from build123d import *

# Parameters (mm, degrees)
CIRPATTERN2_COUNT = 3


with BuildPart() as part:
    # Sketch1 → Base-Revolve (revolve)
    with BuildSketch(Plane.XY):
        with BuildLine():
            Line((-50, 0), (-50, 1.25))
            ThreePointArc((-50, 1.25), (-49.010050505, 7.072345027), (-46.68190465, 12.5))
            Line((-46.68190465, 12.5), (46.650635095, 12.5))
            ThreePointArc((46.650635095, 12.5), (49.148145657, 6.470476128), (50, 0))
            Line((50, 0), (-50, 0))
        make_face()
    revolve(axis=Axis((-57, 0, 0), (1, 0, 0)))

    # Cut-Sweep3: sweep along a path in Sketch3
    with BuildLine(Plane(origin=(0, 0, 0), x_dir=(1, 0, 0), z_dir=(0, 1, 0))) as cut_sweep3_path:
        Line((-16.666666667, -12.5), (-10.416666667, -11.25))
        Line((-10.416666667, -11.25), (10.416666667, -11.25))
        Line((10.416666667, -11.25), (16.666666667, -12.5))
    # Sketch4 → Cut-Sweep3 (sweep, cut)
    with BuildSketch(Plane(origin=(-16.666666667, 0, 0), x_dir=(0, 0, -1), z_dir=(1, 0, 0))):
        Polygon((-12.5, 0), (-14.378358908, 1.315241067), (-14.378358908, -1.315241067), align=None)
    cut_sweep3 = sweep(path=cut_sweep3_path.line, transition=Transition.RIGHT, mode=Mode.SUBTRACT)

    # CirPattern2: Cut-Sweep3 ×3 about axis
    cirpattern2_axis = Axis((0, 0, 0), (1, 0, 0))
    for i in range(1, CIRPATTERN2_COUNT):
        add(cut_sweep3.rotate(cirpattern2_axis, i * 360 / CIRPATTERN2_COUNT), mode=Mode.SUBTRACT)


solid = part.part
Could you check a few things on this model? Use its own coordinates, in mm. Give positions to 0.01 mm unless a question says otherwise; leave off trailing zeros. Order: outer loops, then holes, each group sorted by start corner. A loop starts at its lowest first (then second) coordinate and runs counter-clockwise, first axis right, second up.
1. Suppose I cut it at B-B (y = -6.25). List the corners of the cut face in (x, z) for me, plus the area to 3 significant figures.
2. Suppose I cut it at C-C (z = 0). List the corners of the cut face in (x, y) for me.
3. Will these pins go through, and if not, where does the flat tip stop? P1, Ø5, axis at x = 13.5, z = -7.5, coming from the -Y side; P2, Ø1, axis at x = 3, y = -2, coming from the +Z side; P3, Ø8, axis at x = -28.5, y = 6.5, coming from the -Z side.
4. I need wall thicknesses on L1, parallel to Z at x = -24, y = 0; L2, parallel to X at y = -3.25, z = -9.5; L3, parallel to Z at x = 31.5, y = -3. Which ranges of each line are inside material? Lowest first, please.
5. Suppose I cut it at D-D (x = 37.5). List the corners of the cut face in (y, z) for me.
6. Suppose I cut it at A-A (x = -3). List the corners of the cut face in (y, z) for me (3 decimals).
Solved:
1. outline: (-46.68, -10.83) - (46.65, -10.83) arc R24.21 ccw to (46.65, 10.83) - (-46.68, 10.83) arc R24.21 ccw to start
1. area: 2,100 mm2
2. outline: (-50, -1.25) arc R25 ccw to (-46.68, -12.5) - (46.65, -12.5) arc R25 ccw to (46.65, 12.5) - (-46.68, 12.5) arc R25 ccw to (-50, 1.25) - close
3. P1: stops at y = -11.46
3. P2: stops at z = 12.41
3. P3: stops at z = -12.25
4. L1: z = -12.5 to 12.5
4. L2: x = -47.93 to 47.9
4. L3: z = -12.13 to 12.13
5. outline: circle Ø25 at (0, 0)
6. outline: (-11.234, -5.481) - (-9.743, -5.625) - (-10.364, -6.989) arc R12.5 ccw to (10.364, -6.989) - (9.743, -5.625) - (11.234, -5.481) arc R12.5 ccw to (0.871, 12.47) - (0, 11.25) - (-0.871, 12.47) arc R12.5 ccw to start
